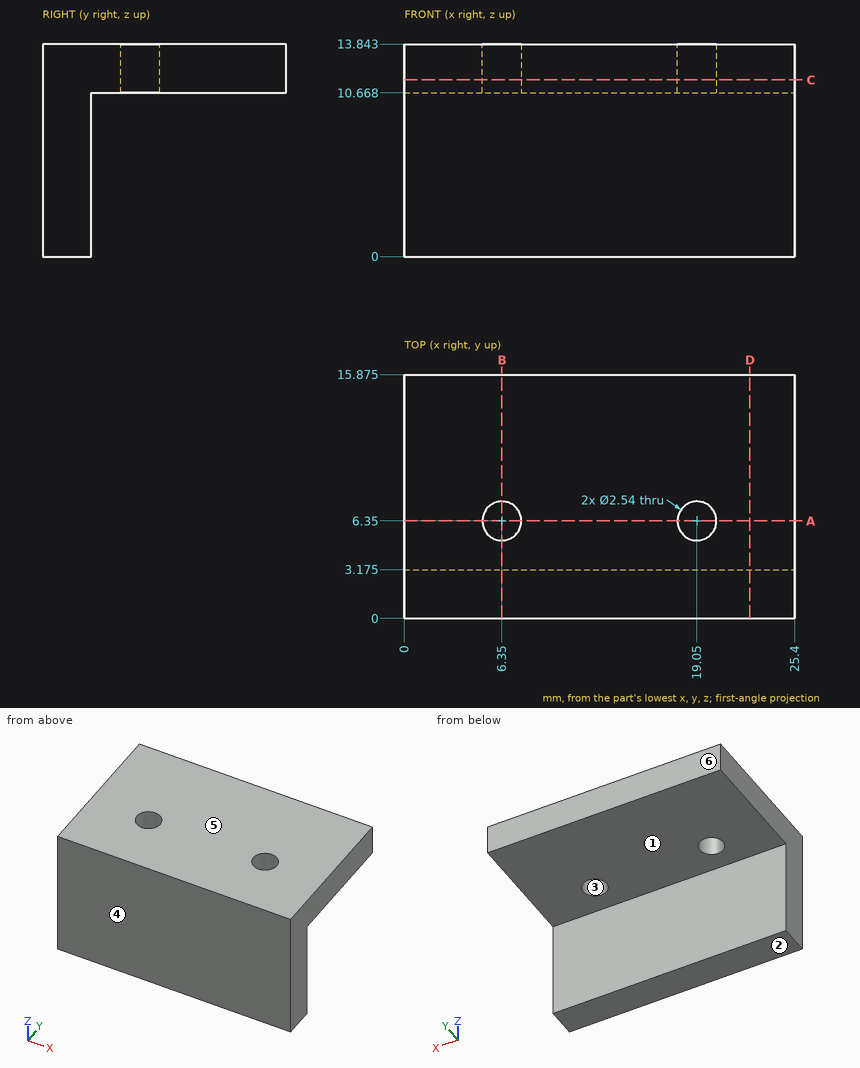
Print and shaded views of the part. All mm, measured from the part's lowest x, y and z. A direction names the side the tool comes from. Coordinates: 2 decimals unless noted, no trailing zeros. Order: outer loops, then holes, each group sorted by start corner. A loop starts at its lowest first (then second) coordinate and runs counter-clockwise, first axis right, second up. Notation, with made-up numbers: (-37.5, -0.75) -> (13.5, -0.75) arc R31 cw to (13.5, 23.25) -> close; hole circle Ø9 at (22, -7.75). An arc over 180 degrees is marked (long way). Use one line per item in the form item = value. Start each with the question number.
1) Drop flat-ended pins along their axis: pin 1 (3 mm diameter, centred on x = 14.5, z = 5.5, fed in from +Y) (3 decimals); pin 2 (6 mm diameter, centred on x = 15.5, y = 8, fed in from -Z). Give the stop position or say it passes through.
2) Tool access for the marked faces 1 and 2: list every direction of +Z, -Z, +X, -X, +Y, -Y with a clear straight run to the whole face (end or side of a thin tool).
3) Band-saw the part on A-A on y = 6.35. Give the cut face in (x, z), then the cut area to 3 significant figures.
4) Pull direction Y, two halves, no side cores. Call the marked faces 3, 4, 5 and 6: +Y half, -Y half, draft (parallel to the pull), parting line (faces both ways), or undercut.
5) Band-saw the part on D-D on x = 22.5. Give the cut face in (y, z) (3 decimals).
6) Band-saw the part on C-C on z = 11.5. Give the cut face in (x, y) (3 decimals).
7) Band-saw the part on B-B on x = 6.35. Give the cut face in (y, z) (3 decimals), then the cut area to 3 significant figures.
8) Drill centre lines: L1, parallel to Y at x = 19.05, z = 11.7 (3 decimals); L2, parallel to Z at x = 15, y = 13; L3, parallel to Y at x = 23.25, z = 6.75 (3 decimals). Where is each one in solid material? Low to high. Write a range as [from, to].
Entries:
q1.pin_1 = 3.175
q1.pin_2 = 10.67
q2.face_1 = -Z, +X, -X, +Y
q2.face_2 = -Z, +X, -X, +Y, -Y
q3.outline = (0, 10.67) -> (5.08, 10.67) -> (5.08, 13.84) -> (0, 13.84) -> close; (7.62, 10.67) -> (17.78, 10.67) -> (17.78, 13.84) -> (7.62, 13.84) -> close; (20.32, 10.67) -> (25.4, 10.67) -> (25.4, 13.84) -> (20.32, 13.84) -> close
q3.area = 64.5 mm2
q4.face_3 = undercut
q4.face_4 = -Y half
q4.face_5 = draft
q4.face_6 = +Y half
q5.outline = (0, 0) -> (3.175, 0) -> (3.175, 10.668) -> (15.875, 10.668) -> (15.875, 13.843) -> (0, 13.843) -> close
q6.outline = (0, 0) -> (25.4, 0) -> (25.4, 15.875) -> (0, 15.875) -> close; hole circle Ø2.54 at (6.35, 6.35); hole circle Ø2.54 at (19.05, 6.35)
q7.outline = (0, 0) -> (3.175, 0) -> (3.175, 10.668) -> (5.08, 10.668) -> (5.08, 13.843) -> (0, 13.843) -> close; (7.62, 10.668) -> (15.875, 10.668) -> (15.875, 13.843) -> (7.62, 13.843) -> close
q7.area = 76.2 mm2
q8.L1 = [0, 5.08], [7.62, 15.875]
q8.L2 = [10.67, 13.84]
q8.L3 = [0, 3.175]
